from build123d import *

# Parameters (mm, degrees)
EXTRUDE047_DEPTH = 3
SKETCH018_R      = 31
EXTRUDE046_DEPTH = 3


with BuildPart() as extrude047:
    # Sketch019 → Extrude047 (new body)
    with BuildSketch(Plane.XY.offset(80)):
        with BuildLine():
            Line((-33, 38), (33, 38))
            ThreePointArc((38, 33), (36.535534, 36.535534), (33, 38))
            Line((38, 33), (38, -33))
            ThreePointArc((33, -38), (36.535534, -36.535534), (38, -33))
            Line((33, -38), (-33, -38))
            ThreePointArc((-38, -33), (-36.535534, -36.535534), (-33, -38))
            Line((-38, -33), (-38, 33))
            ThreePointArc((-33, 38), (-36.535534, 36.535534), (-38, 33))
        make_face()
    extrude(amount=EXTRUDE047_DEPTH)


with BuildPart() as extrude047_1:
    # Extrude047 placement: moved
    add(extrude047.part.moved(Location((0, -3.5, 30))))


with BuildPart() as grill:
    # Sketch018 → Extrude046 (new body)
    with BuildSketch(Plane.XY.offset(80)):
        with BuildLine():
            Line((-34, 39), (34, 39))
            ThreePointArc((39, 34), (37.535534, 37.535534), (34, 39))
            Line((39, 34), (39, -34))
            ThreePointArc((34, -39), (37.535534, -37.535534), (39, -34))
            Line((34, -39), (-34, -39))
            ThreePointArc((-39, -34), (-37.535534, -37.535534), (-34, -39))
            Line((-39, -34), (-39, 34))
            ThreePointArc((-34, 39), (-37.535534, 37.535534), (-39, 34))
        make_face()
        Circle(SKETCH018_R, mode=Mode.SUBTRACT)
    extrude(amount=EXTRUDE046_DEPTH)


with BuildPart() as grill_1:
    # Extrude046 placement: moved
    add(grill.part.moved(Location((0, -3.5, 31))))

    # Cut022: cut Extrude047
    add(extrude047_1.part, mode=Mode.SUBTRACT)


with BuildPart() as grill_2:
    # Cut022 placement: moved
    add(grill_1.part.moved(Location((0, 0, -39))))


solid = grill_2.part
The model under review builds one solid part; all positions refer to its coordinate system, in mm. A direction names the side the tool comes from. Give positions to 0.01 mm unless a question says otherwise; leave off trailing zeros. Write each loop counter-clockwise with the first axis right and the second up, starting at its lowest first coordinate (ties: lowest second). Pieces come first, ordered by that corner, then holes. Notation, with made-up numbers: M 37,50.25 L 68,50.25 A23 ccw 68,89.25 Z; hole C 89,89.25 d8. An arc over 180 degrees is marked long. One line per question, with ' | ' between items. Start each with the question number.
Item 1: Wall thickness on line 1 (X direction, y = -3.5, z = 74.2); line 2 (X direction, y = 28.5, z = 72.35); line 3 (Y direction, x = 22.5, z = 73.9): over which ranges is each line inside the solid? List them lowest first. Write a range as from..to.
Item 2: Draft analysis for pull direction X (two halves, no side actions). For faces 3 (the cylindrical face through (37.5, -41.07, 73.48)), 4 (the cylindrical face through (36.5, -40.07, 72.99)), 5 (the flat face through (-39, -4, 73)), 6 (the flat face through (0, -42.5, 73)), state which applies: released by +X, released by -X, zero draft, split by the parting line, or undercut.
Item 3: We need section A-A on x = 0. Write out the cut boundary in (y, z), plus the area to 3 significant figures.
Item 4: We need section C-C on z = 73.2. Write out the cut boundary in (x, y).
Item 5: For pin 1 (8 mm diameter, centred on x = 28.5, y = 4, fed in from +Z); pin 2 (12 mm diameter, centred on x = 27.5, y = -22.5, fed in from -Z), all flat-tipped, find the tip position at first contact; note any pin that passes through.
Item 6: We need section B-B on y = 18. Write out the cut boundary in (x, z), plus the area to 3 significant figures.
Item 7: For faces 1 (the flat face through (0, 34.5, 73)), 2 (the cylindrical face through (-4.036, 27.236, 74.493)), list the 3-axis set-ups (+Z, -Z, +X, -X, +Y, -Y) from which the entire face can be reached by the end or side of a thin tool; tool diameter is ignored.
Results found:
1) line 1: x = -39..-31, 31..39 | line 2: x = -39..-38, 38..39 | line 3: y = -42.5..-41.5, 34.5..35.5
2) face 3: released by +X | face 4: undercut | face 5: released by -X | face 6: zero draft
3) outline: M -42.5,72 L -41.5,72 L -41.5,74 L -34.5,74 L -34.5,75 L -42.5,75 Z; M 27.5,74 L 34.5,74 L 34.5,72 L 35.5,72 L 35.5,75 L 27.5,75 Z | area: 20.0 mm2
4) outline: M -39,-37.5 A5 ccw -34,-42.5 L 34,-42.5 A5 ccw 39,-37.5 L 39,30.5 A5 ccw 34,35.5 L -34,35.5 A5 ccw -39,30.5 Z; hole M -38,-36.5 A5 ccw -33,-41.5 L 33,-41.5 A5 ccw 38,-36.5 L 38,29.5 A5 ccw 33,34.5 L -33,34.5 A5 ccw -38,29.5 Z
5) pin 1: stops at z = 75 | pin 2: stops at z = 74
6) outline: M -39,72 L -38,72 L -38,74 L -22.33,74 L -22.33,75 L -39,75 Z; M 22.33,74 L 38,74 L 38,72 L 39,72 L 39,75 L 22.33,75 Z | area: 37.3 mm2
7) face 1: -Z | face 2: +Z, -Z
